For this review, take the finished solid that the model builds, in its own axes (mm). A direction names the side the tool comes from. Round coordinates to 2 decimals unless told otherwise and drop trailing zeros. Write each loop counter-clockwise with the first axis right and the second up, starting at its lowest first coordinate (ties: lowest second). Pieces come first, ordered by that corner, then holes. Notation, with made-up numbers: (22.25, -1.5) - (43.25, -1.5) arc R15 cw to (43.25, 25.5) - close; hole circle Ø11 at (54, 63.5). An arc over 180 degrees is marked (long way). One line per item, written item: value. Start each with the question number.
Q1. Mouldability with a two-part tool opening along Y and no side actions: class faces 6 (the face through (67.935, 69, 2)), 7 (the face through (96, 118.24, 2)), 8 (the face through (75, 92.2, 3)) as +Y half, -Y half, draft (parallel to the pull), parting line (faces both ways), or undercut.
Q2. Tool access review of faces 1 (the face through (147.735, 100, 3)), 2 (the face through (125.765, 12.589, 2.465)), 3 (the face through (75, 77.6, 3)), 4 (the face through (143, 128.24, 2)), 5 (the face through (122.335, 13, 2)): name each direction out of +Z, -Z, +X, -X, +Y, -Y from which nothing blocks a thin tool from reaching the whole face with its end or side.
Q3. Add section D-D on y = 96. Write out the cut boundary in (x, z).
Q4. Add section C-C on z = 3.7. Give the number of separate pieces and of enclosed holes in the cut face, and give its area (3 significant figures).
Q5. Add section A-A on y = 83.5. Write out the cut boundary in (x, z).
Q6. Add section B-B on x = 76. Write out the cut boundary in (y, z), and give its area (3 significant figures).
Q7. Clearance check with flat-ended pins moving along their axes: pin 1 Ø1.5 at (y, z) = (38, 4) entering from +X; pin 2 Ø1 at (x, z) = (86.5, 4) entering from -Y; pin 3 Ø0.9 at (x, z) = (75, 4) entering from +Y. State where each tip first meets the part, or that it passes through.
Q8. For probe 1 along Y at (x, z) = (153.5, 3.75); probe 2 along Y at (x, z) = (148, 0.4); probe 3 along X at (y, z) = (13.5, 2.7), list the stretches that pass through material, from the lowest coordinate up.
```python
from build123d import *

# Parameters (mm, degrees)
SKETCH2_W           = 92
SKETCH2_H           = 100
SKETCH2_R           = 3
SKETCH2_W_2         = 2.4
BOSS_EXTRUDE1_DEPTH = 2
BOSS_EXTRUDE3_DEPTH = 3
SKETCH5_W           = 40
SKETCH5_H           = 10
SKETCH5_R           = 1.7
BOSS_EXTRUDE4_DEPTH = 5


with BuildPart() as part:
    # Sketch2 → Boss-Extrude1 (new body)
    # profile 1 of 2: a face of its own
    with BuildSketch(Plane.XY):
        with Locations((113.934873736, 68.240270394)):
            Rectangle(SKETCH2_W, SKETCH2_H)
        with Locations((75.234873736, 39.180270394)):
            Circle(SKETCH2_R, mode=Mode.SUBTRACT)
        with Locations((155.034873736, 36.740270394)):
            Circle(SKETCH2_R, mode=Mode.SUBTRACT)
        with Locations((75.234873736, 84.900270394)):
            Circle(SKETCH2_R, mode=Mode.SUBTRACT)
        with Locations((155.034873736, 100.560270394)):
            Circle(SKETCH2_R, mode=Mode.SUBTRACT)
    # profile 2 of 2: a face of its own
    with BuildSketch(Plane.XY):
        with Locations((161.134873736, 68.240270394)):
            Rectangle(SKETCH2_W_2, SKETCH2_H)
    extrude(amount=BOSS_EXTRUDE1_DEPTH)

    # Sketch3 → Boss-Extrude3 (add)
    with BuildSketch(Plane.XY.offset(2)):
        Polygon((82.534873736, 77.600270394), (67.934873736, 77.600270394), (67.934873736, 46.480270394), (82.534873736, 46.480270394), (82.534873736, 31.880270394), (67.934873736, 31.880270394), (67.934873736, 18.240270394), (162.334873736, 18.240270394), (162.334873736, 29.440270394), (147.734873736, 29.440270394), (147.734873736, 44.040270394), (162.334873736, 44.040270394), (162.334873736, 93.260270394), (147.734873736, 93.260270394), (147.734873736, 107.860270394), (162.334873736, 107.860270394), (162.334873736, 118.240270394), (67.934873736, 118.240270394), (67.934873736, 92.200270394), (82.534873736, 92.200270394), align=None)
    extrude(amount=BOSS_EXTRUDE3_DEPTH)

    # Sketch5 → Boss-Extrude4 (add)
    # profile 1 of 2: a face of its own
    with BuildSketch(Plane(origin=(0, 0, 0), x_dir=(-1, 0, 0), z_dir=(0, 0, -1))):
        with Locations((-142.334873736, 123.240270394)):
            Rectangle(SKETCH5_W, SKETCH5_H)
        with Locations((-157.334873736, 123.240270394)):
            Circle(SKETCH5_R, mode=Mode.SUBTRACT)
        with Locations((-147.334873736, 123.240270394)):
            Circle(SKETCH5_R, mode=Mode.SUBTRACT)
        with Locations((-137.334873736, 123.240270394)):
            Circle(SKETCH5_R, mode=Mode.SUBTRACT)
        with Locations((-127.334873736, 123.240270394)):
            Circle(SKETCH5_R, mode=Mode.SUBTRACT)
    # profile 2 of 2: a face of its own
    with BuildSketch(Plane(origin=(0, 0, 0), x_dir=(-1, 0, 0), z_dir=(0, 0, -1))):
        with Locations((-142.334873736, 13.240270394)):
            Rectangle(SKETCH5_W, SKETCH5_H)
        with Locations((-157.334873736, 13.240270394)):
            Circle(SKETCH5_R, mode=Mode.SUBTRACT)
        with Locations((-147.334873736, 13.240270394)):
            Circle(SKETCH5_R, mode=Mode.SUBTRACT)
        with Locations((-137.334873736, 13.240270394)):
            Circle(SKETCH5_R, mode=Mode.SUBTRACT)
        with Locations((-127.334873736, 13.240270394)):
            Circle(SKETCH5_R, mode=Mode.SUBTRACT)
    extrude(amount=-BOSS_EXTRUDE4_DEPTH)


solid = part.part
```
Result set:
1. face 6: draft
1. face 7: +Y half
1. face 8: undercut
2. face 1: +Z, +X
2. face 2: +Z, -Z
2. face 3: +Z, -X
2. face 4: +Z, -Z, +X, -X, +Y
2. face 5: +Z, -Z, -X, -Y
3. outline: (67.93, 0) - (162.33, 0) - (162.33, 2) - (147.73, 2) - (147.73, 5) - (67.93, 5) - close
4. separate pieces: 1
4. enclosed holes: 8
4. area: 9,310 mm^2
5. outline: (67.93, 0) - (72.58, 0) - (72.58, 2) - (67.93, 2) - close; (77.89, 0) - (162.33, 0) - (162.33, 5) - (82.53, 5) - (82.53, 2) - (77.89, 2) - close
6. outline: (18.24, 0) - (36.28, 0) - (36.28, 2) - (31.88, 2) - (31.88, 5) - (18.24, 5) - close; (42.08, 0) - (82, 0) - (82, 2) - (77.6, 2) - (77.6, 5) - (46.48, 5) - (46.48, 2) - (42.08, 2) - close; (87.8, 0) - (118.24, 0) - (118.24, 5) - (92.2, 5) - (92.2, 2) - (87.8, 2) - close
6. area: 389 mm^2
7. pin 1: stops at x = 147.73
7. pin 2: stops at y = 18.24
7. pin 3: stops at y = 118.24
8. probe 1: y = 8.24 to 29.44, 44.04 to 93.26, 107.86 to 128.24
8. probe 2: y = 8.24 to 11.68, 14.8 to 121.68, 124.8 to 128.24
8. probe 3: x = 122.33 to 125.65, 129.01 to 135.65, 139.01 to 145.65, 149.01 to 155.65, 159.01 to 162.33
